Source: CAD feature listing. Evaluate the final solid. Frame: model axes, mm. Give positions to 0.01 mm unless a question says otherwise; leave off trailing zeros. Order: outer loops, then holes, each group sorted by start corner. A loop starts at its lowest first (then second) coordinate and runs counter-clockwise, first axis right, second up. Notation, with made-up numbers: (-10, 0.25) - (-2, 0.25) arc R37 ccw to (-2, 38.25) - close; hole circle Ø10 at (9.5, -28). An arc over 180 degrees is marked (long way). Use CSV: the item, a comma, the result in double quotes.
```python
from build123d import *

# Parameters (mm, degrees)
ESQUISSE1_W             = 40
ESQUISSE1_H             = 54
BOSS_EXTRU_1_DEPTH      = 4
ESQUISSE2_W             = 46
ESQUISSE2_H             = 60
BOSS_EXTRU_2_DEPTH      = 2
CONG_1_R                = 4
ESQUISSE3_R             = 1
ENL_V_MAT_EXTRU_1_DEPTH = 76.709972923


with BuildPart() as part:
    # Esquisse1 → Boss.-Extru.1 (new body)
    with BuildSketch(Plane.XY):
        with Locations((23, 30)):
            Rectangle(ESQUISSE1_W, ESQUISSE1_H)
    extrude(amount=BOSS_EXTRU_1_DEPTH)

    # Esquisse2 → Boss.-Extru.2 (add)
    with BuildSketch(Plane.XY):
        with Locations((23, 30)):
            Rectangle(ESQUISSE2_W, ESQUISSE2_H)
    extrude(amount=BOSS_EXTRU_2_DEPTH)

    # Congé1
    cong_1_edges = [part.edges().sort_by_distance(p)[0] for p in [
        (0, 60, 1),
        (0, 0, 1),
        (46, 0, 1),
        (46, 60, 1),
    ]]
    fillet(cong_1_edges, radius=CONG_1_R)

    # Esquisse3 → Enlèv. mat.-Extru.1 (cut, through all)
    with BuildSketch(Plane.XY):
        with Locations((44.5, 5)):
            Circle(ESQUISSE3_R)
        with Locations((1.5, 5)):
            Circle(ESQUISSE3_R)
        with Locations((1.5, 55)):
            Circle(ESQUISSE3_R)
        with Locations((44.5, 55)):
            Circle(ESQUISSE3_R)
    extrude(amount=ENL_V_MAT_EXTRU_1_DEPTH, mode=Mode.SUBTRACT)


solid = part.part
```
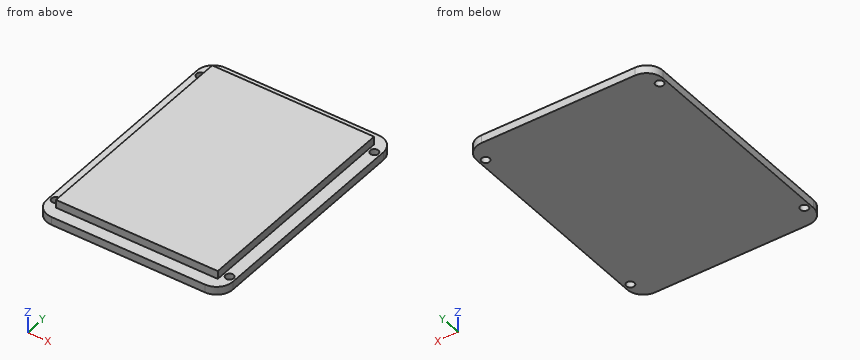
Item 1: First-contact query: pin 1 (1 mm diameter, centred on y = 21.5, z = 3.5, fed in from +X); pin 2 (1 mm diameter, centred on x = 9.5, z = 3, fed in from -Y); pin 3 (1.6 mm diameter, centred on x = 23, z = 3, fed in from +Y). Flat tips, straight axial feed; report the tip coordinate or a pass-through.
Filled in:
pin 1,"stops at x = 43"
pin 2,"stops at y = 3"
pin 3,"stops at y = 57"
Item 2: Section B-B on x = 17.5. Return the cut outline in (y, z), then the cut area to 3 significant figures.
Filled in:
outline,"(0, 0) - (60, 0) - (60, 2) - (57, 2) - (57, 4) - (3, 4) - (3, 2) - (0, 2) - close"
area,"228 mm2"
Item 3: Section C-C on y = 37.5. Return the cut outline in (x, z), then the cut area to 3 significant figures.
Filled in:
outline,"(0, 0) - (46, 0) - (46, 2) - (43, 2) - (43, 4) - (3, 4) - (3, 2) - (0, 2) - close"
area,"172 mm2"
Item 4: Material intervals for line 1 (X direction, y = 55, z = 1.4); line 2 (Y direction, x = 1.5, z = 1.45); line 3 (X direction, y = 8.5, z = 2.65), sorted ascending. Write a range as from..to.
Filled in:
line 1,"x = 0..0.5, 2.5..43.5, 45.5..46"
line 2,"y = 0.88..4, 6..54, 56..59.12"
line 3,"x = 3..43"
Item 5: Section D-D on x = 44.5. Return the cut outline in (y, z), then the cut area to 3 significant figures.
Filled in:
outline,"(0.88, 0) - (4, 0) - (4, 2) - (0.88, 2) - close; (6, 0) - (54, 0) - (54, 2) - (6, 2) - close; (56, 0) - (59.12, 0) - (59.12, 2) - (56, 2) - close"
area,"108 mm2"
Item 6: Section A-A on y = 5. Return the cut outline in (x, z).
Filled in:
outline,"(0, 0) - (0.5, 0) - (0.5, 2) - (0, 2) - close; (2.5, 0) - (43.5, 0) - (43.5, 2) - (43, 2) - (43, 4) - (3, 4) - (3, 2) - (2.5, 2) - close; (45.5, 0) - (46, 0) - (46, 2) - (45.5, 2) - close"
